```python
from build123d import *

# Parameters (mm, degrees)
F1_DEPTH       = 2
F2_DEPTH       = 4
F3_R           = 1.99999
F4_D           = 3.3
F4_CSINK_D     = 8.96
F4_CSINK_ANGLE = 90


# Not quite as in the source:
# - a fillet or chamfer is up to 0.001 mm smaller than in the source, because OpenCascade refuses the exact size


with BuildPart() as f1:
    # F0 (on Top) → F1 (new body)
    with BuildSketch(Plane.XY):
        with BuildLine():
            Line((32.5, 26.9999996311), (-32.5, 26.9999996311))
            ThreePointArc((-32.5, 26.9999996311), (-37.4497472074, 24.9497472074), (-39.4999996311, 20))
            Line((-39.4999996311, 20), (-39.4999996311, -20))
            ThreePointArc((-39.4999996311, -20), (-37.4497472074, -24.9497472074), (-32.5, -26.9999996311))
            Line((-32.5, -26.9999996311), (32.5, -26.9999996311))
            ThreePointArc((32.5, -26.9999996311), (37.4497472074, -24.9497472074), (39.4999996311, -20))
            Line((39.4999996311, -20), (39.4999996311, 20))
            ThreePointArc((39.4999996311, 20), (37.4497472074, 24.9497472074), (32.5, 26.9999996311))
        make_face()
        with BuildLine():
            ThreePointArc((-37.5, 20), (-36.0355339059, 23.5355339059), (-32.5, 25))
            Line((-32.5, 25), (32.5, 25))
            ThreePointArc((32.5, 25), (36.0355339059, 23.5355339059), (37.5, 20))
            Line((37.5, 20), (37.5, -20))
            ThreePointArc((37.5, -20), (36.0355339059, -23.5355339059), (32.5, -25))
            Line((32.5, -25), (-32.5, -25))
            ThreePointArc((-32.5, -25), (-36.0355339059, -23.5355339059), (-37.5, -20))
            Line((-37.5, -20), (-37.5, 20))
        make_face(mode=Mode.SUBTRACT)
        with BuildLine():
            Line((32.5, 25), (-32.5, 25))
            ThreePointArc((-32.5, 25), (-36.0355339059, 23.5355339059), (-37.5, 20))
            Line((-37.5, 20), (-37.5, -20))
            ThreePointArc((-37.5, -20), (-36.0355339059, -23.5355339059), (-32.5, -25))
            Line((-32.5, -25), (32.5, -25))
            ThreePointArc((32.5, -25), (36.0355339059, -23.5355339059), (37.5, -20))
            Line((37.5, -20), (37.5, 20))
            ThreePointArc((37.5, 20), (36.0355339059, 23.5355339059), (32.5, 25))
        make_face()
    extrude(amount=F1_DEPTH)

    # F0 (on Top) → F2 (join)
    with BuildSketch(Plane.XY):
        with BuildLine():
            Line((32.5, 25), (-32.5, 25))
            ThreePointArc((-32.5, 25), (-36.0355339059, 23.5355339059), (-37.5, 20))
            Line((-37.5, 20), (-37.5, -20))
            ThreePointArc((-37.5, -20), (-36.0355339059, -23.5355339059), (-32.5, -25))
            Line((-32.5, -25), (32.5, -25))
            ThreePointArc((32.5, -25), (36.0355339059, -23.5355339059), (37.5, -20))
            Line((37.5, -20), (37.5, 20))
            ThreePointArc((37.5, 20), (36.0355339059, 23.5355339059), (32.5, 25))
        make_face()
    extrude(amount=F2_DEPTH)

    # F3 (radius 2 in the source; OpenCascade refuses exactly that, so slightly less here)
    f3_edges = [f1.edges().sort_by_distance(p)[0] for p in [
        (0, 27, 0),
        (-37.449747, 24.949747, 0),
        (-39.5, 0, 0),
        (-37.449747, -24.949747, 0),
        (0, -27, 0),
        (37.449747, -24.949747, 0),
        (39.5, 0, 0),
        (37.449747, 24.949747, 0),
    ]]
    fillet(f3_edges, radius=F3_R)

    # F4 (through all)
    with Locations(Plane(origin=(0, 0, 0), x_dir=(1, 0, 0), z_dir=(0, 0, -1))):
        with Locations((32.5, 20), (32.5, -20), (-32.5, -20), (-32.5, 20)):
            CounterSinkHole(F4_D / 2, F4_CSINK_D / 2, counter_sink_angle=F4_CSINK_ANGLE)


solid = f1.part
```
Source: CAD feature listing. Evaluate the final solid. Frame: model axes, mm. A direction names the side the tool comes from. Round coordinates to 2 decimals unless told otherwise and drop trailing zeros. Loops run counter-clockwise (first coordinate to the right, second up) from the corner with the lowest first, then second, coordinate; pieces in that order, holes last. Notation, with made-up numbers: M 53.5,65.5 L 70.5,65.5 A36 ccw 70.5,104.5 Z; hole C -38,85.25 d9. An arc over 180 degrees is marked long. Put each result on its own line as item: value.
(1) Ray query, line 1 (X direction, y = 20, z = 3.25); line 2 (Y direction, x = 32.5, z = 3.4); line 3 (Y direction, x = 30, z = 0.65). Return the intervals inside material, ascending. Write a range as [from, to].
Solutions:
line 1: [-37.5, -34.15], [-30.85, 30.85], [34.15, 37.5]
line 2: [-25, -21.65], [-18.35, 18.35], [21.65, 25]
line 3: [-26.48, -22.9], [-17.1, 17.1], [22.9, 26.48]
(2) Pull-direction query (Y, two-part tool) for faces 1 (the face through (-30.71, 19.92, 2.69)), 2 (the face through (-1, 0, 4)), 3 (the face through (0, -25, 3)); classes: released by +Y, released by -Y, zero draft, split by the parting line, or undercut.
Solutions:
face 1: undercut
face 2: zero draft
face 3: released by -Y
(3) Section A-A, the plane z = 0.85. Return loops of the section in (x, y), and give its area (3 significant figures).
Solutions:
outline: M -39.14,-20 A6.64 ccw -32.5,-26.64 L 32.5,-26.64 A6.64 ccw 39.14,-20 L 39.14,20 A6.64 ccw 32.5,26.64 L -32.5,26.64 A6.64 ccw -39.14,20 Z; hole C -32.5,-20 d7.26; hole C -32.5,20 d7.26; hole C 32.5,-20 d7.26; hole C 32.5,20 d7.26
area: 3,970 mm²
(4) Access query for faces 4 (the face through (-36, 23.57, 2.99)), 5 (the face through (37.5, 0, 3)), 6 (the face through (0, -26, 2)), 7 (the face through (36, -23.57, 2.99)), 8 (the face through (-37.5, 0, 3)). Directions: +Z, -Z, +X, -X, +Y, -Y. A direction counts if a zero-diameter tool reaches every point of the face in a straight line with its end or side. Return the directions, or none.
Solutions:
face 4: +Z, -X, +Y
face 5: +Z, +X, +Y, -Y
face 6: +Z
face 7: +Z, +X, -Y
face 8: +Z, -X, +Y, -Y
(5) First-contact query: pin 1 (1.5 mm diameter, centred on y = 15, z = 3, fed in from -X); pin 2 (1 mm diameter, centred on x = 0, z = 0.5, fed in from +Y); pin 3 (0.6 mm diameter, centred on x = -5, z = 3, fed in from -Y). Flat tips, straight axial feed; report the tip coordinate or a pass-through.
Solutions:
pin 1: x = -37.5
pin 2: y = 26.73
pin 3: y = -25
